Geometry: final body of the model. Coordinates: model frame, mm. Face numbers are marked on the shaded views. Give positions to 0.01 mm unless a question says otherwise; leave off trailing zeros. Loops run counter-clockwise (first coordinate to the right, second up) from the corner with the lowest first, then second, coordinate; pieces in that order, holes last.
1. Section A-A, the plane z = -19.05. Output: boundary loops of the cut face in (x, y) (3 decimals), then the cut area to 3 significant figures.
2. First-contact query: P1, Ø6.5, axis at x = 56.5, z = -17, coming from the -Y side. Flat tip, straight axial feed; report the tip coordinate or a pass-through.
3. Draft query along Z for the marked faces 1, 2 and 3. Return one class per face: +Z half, -Z half, draft (parallel to the pull), parting line (faces both ways), or undercut.
4. Section B-B, the plane x = 57.15. Output: boundary loops of the cut face in (y, z) (3 decimals).
5. Material intervals for line 1 along Z through (x, y) = (57.15, 2.25); line 2 along Z through (x, y) = (57.15, 5) (3 decimals); line 3 along X through (y, z) = (1.5, -24), sorted ascending.
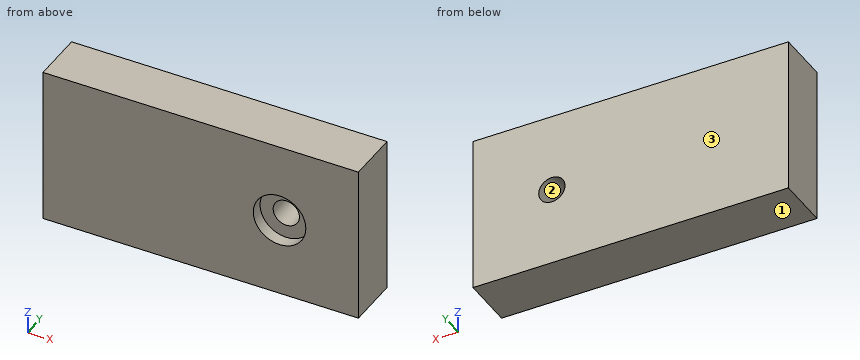
from build123d import *

# Parameters (mm, degrees)
SKETCH1_W           = 76.2
SKETCH1_H           = 38.1
BOSS_EXTRUDE1_DEPTH = 12.7
SKETCH2_R           = 3.175
CUT_EXTRUDE1_DEPTH  = 13.7
SKETCH3_R           = 6.35
CUT_EXTRUDE2_DEPTH  = 3


with BuildPart() as part:
    # Sketch1 → Boss-Extrude1 (new body)
    with BuildSketch(Plane(origin=(0, 0, 0), x_dir=(1, 0, 0), z_dir=(0, 1, 0))):
        with Locations((38.1, 19.05)):
            Rectangle(SKETCH1_W, SKETCH1_H)
    extrude(amount=BOSS_EXTRUDE1_DEPTH)

    # Sketch2 → Cut-Extrude1 (cut, through all)
    with BuildSketch(Plane.XZ):
        with Locations((57.15, -19.05)):
            Circle(SKETCH2_R)
    extrude(amount=-CUT_EXTRUDE1_DEPTH, mode=Mode.SUBTRACT)

    # Sketch3 → Cut-Extrude2 (cut)
    with BuildSketch(Plane.XZ):
        with Locations((57.15, -19.05)):
            Circle(SKETCH3_R)
    extrude(amount=-CUT_EXTRUDE2_DEPTH, mode=Mode.SUBTRACT)


solid = part.part
Answers below:
1. outline: (0, 0) - (50.8, 0) - (50.8, 3) - (53.975, 3) - (53.975, 12.7) - (0, 12.7) - close; (60.325, 3) - (63.5, 3) - (63.5, 0) - (76.2, 0) - (76.2, 12.7) - (60.325, 12.7) - close
1. area: 868 mm2
2. P1: stops at y = 3
3. face 1: -Z half
3. face 2: undercut
3. face 3: draft
4. outline: (0, -38.1) - (12.7, -38.1) - (12.7, -22.225) - (3, -22.225) - (3, -25.4) - (0, -25.4) - close; (0, -12.7) - (3, -12.7) - (3, -15.875) - (12.7, -15.875) - (12.7, 0) - (0, 0) - close
5. line 1: z = -38.1 to -25.4, -12.7 to 0
5. line 2: z = -38.1 to -22.225, -15.875 to 0
5. line 3: x = 0 to 53.17, 61.13 to 76.2
